CAD build for the part. Positions are in the model's coordinates, mm. A direction names the side the tool comes from. Give positions to 0.01 mm unless a question says otherwise; leave off trailing zeros. Write each loop counter-clockwise with the first axis right and the second up, starting at its lowest first coordinate (ties: lowest second). Pieces come first, ordered by that corner, then holes. Notation, with made-up numbers: (-32.5, -0.75) -> (-16.5, -0.75) arc R32 ccw to (-16.5, 28.25) -> close; hole circle Ø2 at (-26.75, 13.5). An arc over 180 degrees is marked (long way). Answer as a JSON object with one key per item and string values.
```python
from build123d import *

# Parameters (mm, degrees)
SKETCH1_R           = 50.8
BOSS_EXTRUDE1_DEPTH = 50.8
SKETCH3_R           = 3.175
CUT_EXTRUDE1_DEPTH  = 6.35
CIRPATTERN1_COUNT   = 4
CUT_EXTRUDE2_DEPTH  = 6.35
CUT_EXTRUDE3_START  = 2.54
CUT_EXTRUDE3_DEPTH  = 2.54
CIRPATTERN2_COUNT   = 4
SKETCH6_R           = 12.7
CUT_EXTRUDE4_DEPTH  = 88.988181024


with BuildPart() as part:
    # Sketch1 → Boss-Extrude1 (new body)
    with BuildSketch(Plane(origin=(0, 0, 0), x_dir=(1, 0, 0), z_dir=(0, 1, 0))):
        with Locations(Location((0, 0, 0), (0, 0, 270))):
            Circle(SKETCH1_R)
    extrude(amount=BOSS_EXTRUDE1_DEPTH)

    # Sketch3 → Cut-Extrude1 (cut)
    with BuildSketch(Plane.XZ):
        with Locations(Location((0, 44.45, 0), (0, 0, 270))):
            Circle(SKETCH3_R)
    cut_extrude1 = extrude(amount=-CUT_EXTRUDE1_DEPTH, mode=Mode.SUBTRACT)

    # CirPattern1: Cut-Extrude1 ×4 about axis
    cirpattern1_axis = Axis((0, 0, 0), (0, 1, 0))
    for i in range(1, CIRPATTERN1_COUNT):
        add(cut_extrude1.rotate(cirpattern1_axis, i * 360 / CIRPATTERN1_COUNT), mode=Mode.SUBTRACT)

    # Sketch4 → Cut-Extrude2 (cut)
    with BuildSketch(Plane.XZ):
        with BuildLine():
            Line((43.18, -4.731127947), (43.18, -2.909935566))
            ThreePointArc((43.18, -2.909935566), (44.45, -3.175), (45.72, -2.909935566))
            Line((45.72, -2.909935566), (45.72, -4.731127947))
            ThreePointArc((45.72, -4.731127947), (44.45, -4.898619361), (43.18, -4.731127947))
        make_face()
    cut_extrude2 = extrude(amount=-CUT_EXTRUDE2_DEPTH, mode=Mode.SUBTRACT)

    # Sketch5 → Cut-Extrude3 (cut)
    with BuildSketch(Plane.XZ.offset(-6.35).offset(CUT_EXTRUDE3_START)):
        with BuildLine():
            Line((47.625, 0), (49.348619361, 0))
            ThreePointArc((49.348619361, 0), (48.337011592, -2.98120991), (45.72, -4.731127947))
            Line((45.72, -4.731127947), (45.72, -2.909935566))
            ThreePointArc((45.72, -2.909935566), (47.106395584, -1.73901912), (47.625, 0))
        make_face()
    cut_extrude3 = extrude(amount=-CUT_EXTRUDE3_DEPTH, mode=Mode.SUBTRACT)

    # CirPattern2: Cut-Extrude2, Cut-Extrude3 ×4 about axis
    cirpattern2_axis = Axis((0, 0, 0), (0, 1, 0))
    add([cut_extrude2.rotate(cirpattern2_axis, i * 360 / CIRPATTERN2_COUNT) for i in range(1, CIRPATTERN2_COUNT)], mode=Mode.SUBTRACT)
    add([cut_extrude3.rotate(cirpattern2_axis, i * 360 / CIRPATTERN2_COUNT) for i in range(1, CIRPATTERN2_COUNT)], mode=Mode.SUBTRACT)

    # Sketch6 → Cut-Extrude4 (cut, through all)
    with BuildSketch(Plane(origin=(0, 50.8, 0), x_dir=(1, 0, 0), z_dir=(0, 1, 0))):
        with Locations(Location((0, 0, 0), (0, 0, 270))):
            Circle(SKETCH6_R)
    extrude(amount=-CUT_EXTRUDE4_DEPTH, mode=Mode.SUBTRACT)


solid = part.part
```
1) Slice it at A-A (x = 7). List the corners of the cut face in (y, z), then the cut area to 3 significant figures.
Model answer:
{"outline": "(0, -50.32) -> (50.8, -50.32) -> (50.8, -10.6) -> (0, -10.6) -> close; (0, 10.6) -> (50.8, 10.6) -> (50.8, 50.32) -> (0, 50.32) -> close", "area": "4,040 mm2"}
2) Slice it at D-D (z = 23.5). List the corners of the cut face in (x, y).
Model answer:
{"outline": "(-45.04, 0) -> (45.04, 0) -> (45.04, 50.8) -> (-45.04, 50.8) -> close"}
3) Slice it at C-C (x = 44.45). List the corners of the cut face in (y, z) (3 decimals), then the cut area to 3 significant figures.
Model answer:
{"outline": "(0, -24.593) -> (50.8, -24.593) -> (50.8, 24.593) -> (0, 24.593) -> (0, 3.175) -> (6.35, 3.175) -> (6.35, -4.899) -> (0, -4.899) -> close", "area": "2,450 mm2"}
4) Mould opens along Z. For faces 4 (the cylindrical face through (-30.911, 25.044, -40.313)), 5 (the flat face through (48, 3.81, -2)), 6 (the flat face through (-11, 0, 11)) say: released by +Z, released by -Z, zero draft, split by the parting line, or undercut.
Model answer:
{"face 4": "split by the parting line", "face 5": "undercut", "face 6": "zero draft"}
5) Slice it at B-B (y = 19). List the corners of the cut face in (x, z).
Model answer:
{"outline": "circle Ø101.6 at (0, 0); hole circle Ø25.4 at (0, 0)"}
6) 3-axis set-ups, long thin cutter, end or side, ignore diameter. For faces 1 (the flat face through (1, 6.35, 45)), 2 (the cylindrical face through (42.741, 3.131, 2.676)), 3 (the flat face through (-11, 50.8, 11)): which of +Z, -Z, +X, -X, +Y, -Y reach the whole face in a straight line?
Model answer:
{"face 1": "none", "face 2": "-Y", "face 3": "+Z, -Z, +X, -X, +Y"}
7) Pin check, flat tips, straight feed: pin 1 (1.5 mm diameter, centred on y = 2, z = -3.5, fed in from -X); pin 2 (2 mm diameter, centred on x = -25.5, y = 11.5, fed in from +Z); pin 3 (10 mm diameter, centred on x = 5.5, z = 8.5, fed in from -Y); pin 4 (2 mm diameter, centred on y = 3.5, z = -4.5, fed in from +X). Stop position of each tip, or through.
Model answer:
{"pin 1": "stops at x = -50.73", "pin 2": "stops at z = 44.5", "pin 3": "stops at y = 0", "pin 4": "stops at x = 50.68"}
8) Wall check: probe 1 along X at (y, z) = (37, 0); probe 2 along X at (y, z) = (2.25, 0) (3 decimals); probe 3 along X at (y, z) = (46.5, -10). Give the ranges that are in metal, low to high.
Model answer:
{"probe 1": "x = -50.8 to -12.7, 12.7 to 50.8", "probe 2": "x = -50.8 to -47.625, -41.275 to -12.7, 12.7 to 41.275, 47.625 to 50.8", "probe 3": "x = -49.81 to -7.83, 7.83 to 49.81"}
